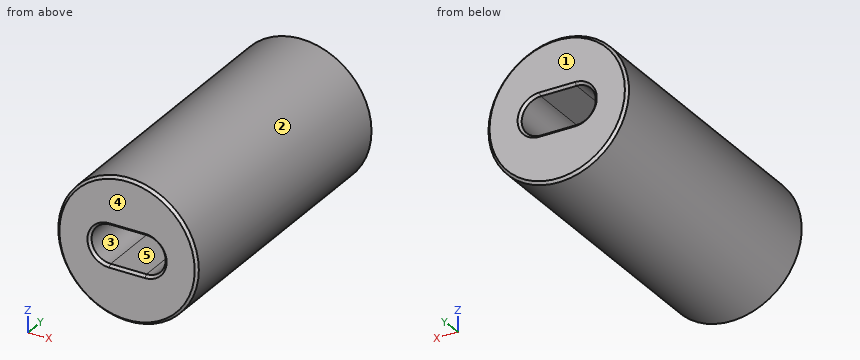
from build123d import *

# Parameters (mm, degrees)
SKETCH1_R          = 2.75
SKETCH1_R_2        = 1.45
MAIN_EXTRUDE_DEPTH = 5.7
MAIN_CHAMFER_SIZE  = 0.1


with BuildPart() as part:
    # Sketch1 → main extrude (new body, symmetric)
    with BuildSketch(Plane(origin=(0, 0, 0), x_dir=(1, 0, 0), z_dir=(0, 1, 0))):
        Circle(SKETCH1_R)
        Circle(SKETCH1_R_2, mode=Mode.SUBTRACT)
        with BuildLine():
            ThreePointArc((-0.7, -0.75), (-1.230330086, -0.530330086), (-1.45, 0))
            ThreePointArc((-1.45, 0), (0, -1.45), (1.45, 0))
            ThreePointArc((1.45, 0), (1.230330086, -0.530330086), (0.7, -0.75))
            Line((0.7, -0.75), (-0.7, -0.75))
        make_face()
        with BuildLine():
            ThreePointArc((-1.45, 0), (-1.230330086, 0.530330086), (-0.7, 0.75))
            Line((-0.7, 0.75), (0.7, 0.75))
            ThreePointArc((0.7, 0.75), (1.230330086, 0.530330086), (1.45, 0))
            ThreePointArc((1.45, 0), (0, 1.45), (-1.45, 0))
        make_face()
    extrude(amount=MAIN_EXTRUDE_DEPTH, both=True)

    # main chamfer
    main_chamfer_edges = [part.edges().sort_by_distance(p)[0] for p in [
        (0, 5.7, 0.75),
        (-1.45, 5.7, 0),
        (-2.75, 5.7, 0),
        (0, 5.7, -0.75),
        (-2.75, -5.7, 0),
        (-1.45, -5.7, 0),
        (0, -5.7, 0.75),
        (1.45, -5.7, 0),
        (0, -5.7, -0.75),
        (1.45, 5.7, 0),
    ]]
    chamfer(main_chamfer_edges, length=MAIN_CHAMFER_SIZE)


solid = part.part
Source: CAD feature listing. Evaluate the final solid. Frame: model axes, mm. Face numbers are marked on the shaded views. A direction names the side the tool comes from. Give positions to 0.01 mm unless a question says otherwise; leave off trailing zeros. Order: outer loops, then holes, each group sorted by start corner. A loop starts at its lowest first (then second) coordinate and runs counter-clockwise, first axis right, second up. Notation, with made-up numbers: (58, 44.5) -> (112, 44.5) arc R13 ccw to (112, 55.5) -> close; hole circle Ø8 at (20, 83). An arc over 180 degrees is marked (long way). Write item = value, one per line.
Item 1: Contact query for flat-ended pins moving along their axis: pin 1 (1.5 mm diameter, centred on y = -2.5, z = -1, fed in from +X); pin 2 (1 mm diameter, centred on x = -1.5, y = 0, fed in from +Z). Output: stop coordinate, or through.
Check result:
pin_1 = 2.74
pin_2 = 2.56
Item 2: Section query A-A (x = 0). Output: boundary loops of the cut face in (y, z), then the cut area to 3 significant figures.
Check result:
outline = (-5.7, -2.65) -> (-5.6, -2.75) -> (5.6, -2.75) -> (5.7, -2.65) -> (5.7, -0.85) -> (5.6, -0.75) -> (-5.6, -0.75) -> (-5.7, -0.85) -> close; (-5.7, 0.85) -> (-5.6, 0.75) -> (5.6, 0.75) -> (5.7, 0.85) -> (5.7, 2.65) -> (5.6, 2.75) -> (-5.6, 2.75) -> (-5.7, 2.65) -> close
area = 45.6 mm²
Item 3: Section query B-B (y = 4.5). Output: boundary loops of the cut face in (x, z), then the cut area to 3 significant figures.
Check result:
outline = circle Ø5.5 at (0, 0); hole (-0.7, -0.75) -> (0.7, -0.75) arc R0.75 ccw to (0.7, 0.75) -> (-0.7, 0.75) arc R0.75 ccw to start
area = 19.9 mm²
Item 4: Set-up query: the marked faces 4 and 5. Return all of +Z, -Z, +X, -X, +Y, -Y with unobstructed straight access to the full face (end or side cutting, diameter ignored); none if empty.
Check result:
face_4 = +Z, -Z, +X, -X, -Y
face_5 = +Y, -Y
Item 5: Ray query, probe 1 along X at (y, z) = (-3.5, 0); probe 2 along X at (y, z) = (1.5, 0.4); probe 3 along Z at (x, y) = (-1.2, 2.25). Return the intervals inside material, ascending.
Check result:
probe_1 = -2.75 to -1.45, 1.45 to 2.75
probe_2 = -2.72 to -1.33, 1.33 to 2.72
probe_3 = -2.47 to -0.56, 0.56 to 2.47
Item 6: Mould query, pull axis X, two halves, no side actions, for the marked faces 1, 2 and 3. Classes: +X half, -X half, draft (parallel to the pull), parting line (faces both ways), or undercut.
Check result:
face_1 = draft
face_2 = parting line
face_3 = undercut
